Check sheet for the modelled part. Datum: model origin and axes. Units: mm. A direction names the side the tool comes from. Coordinates: 2 decimals unless noted, no trailing zeros. Loops run counter-clockwise (first coordinate to the right, second up) from the corner with the lowest first, then second, coordinate; pieces in that order, holes last. Notation, with made-up numbers: (20.25, 78) - (58.25, 78) arc R14 cw to (58.25, 103) - close; hole circle Ø1 at (-24.75, -37.5). An arc over 180 degrees is marked (long way). Write each question's results on one line, items separated by ' | '. Start each with the question number.
1. Cross-section at A-A (z = 59.5). Record the cut outline in (x, y).
2. Cross-section at B-B (y = -4.5). Record the cut outline in (x, z).
3. Draft check along X on faces 1 (the face through (-236, -11, 2)), 2 (the face through (-257, -1, 67.38)). Enter one of: released by +X, released by -X, zero draft, split by the parting line, or undercut.
4. Gauge pin test, flat end, axial feed: P1, Ø2.5, axis at x = -276.61, y = 6.8, coming from the +Z side. Record the tip position at first contact, or that the pin passes through.
5. Thickness scan on line 1 (Z direction, x = -234.5, y = -9); line 2 (Y direction, x = -240.5, z = 19); line 3 (Z direction, x = -234, y = 12). Record the ranges inside material, lowest first. Write a range as [from, to].
6. Tool access check on faces 3 (the face through (-257, -1, 0)), 4 (the face through (-257, -17.196, 33)), 5 (the face through (-235.52, 4.3, 64.37)). Record the directions out of +Z, -Z, +X, -X, +Y, -Y that give a thin tool (end or side, any length) a straight path to the whole face; none if there is none.
7. Cross-section at C-C (x = -271.5). Record the cut outline in (y, z).
```python
from build123d import *

# Parameters (mm, degrees)
SKETCH1_W               = 55.67262225
SKETCH1_H               = 40
BOSS_EXTRUDE1_DEPTH     = 4
SKETCH2_W               = 55.67262225
SKETCH2_H               = 4
BOSS_EXTRUDE2_DEPTH     = 63.38
SKETCH3_W               = 55.67262225
SKETCH3_H               = 40
BOSS_EXTRUDE3_DEPTH     = 4
SKETCH4_R               = 1.6
CUT_EXTRUDE1_DEPTH      = 64.38
CUT_EXTRUDE1_DEPTH_BACK = 5
CUT_EXTRUDE2_START      = -2
CUT_EXTRUDE2_DEPTH      = 63.38
FILLET1_R               = 3


with BuildPart() as part:
    # Sketch1 → Boss-Extrude1 (new body)
    with BuildSketch(Plane.XY):
        with Locations((-256.769960814, -1.19608299)):
            Rectangle(SKETCH1_W, SKETCH1_H)
    extrude(amount=BOSS_EXTRUDE1_DEPTH)

    # Sketch2 → Boss-Extrude2 (add)
    with BuildSketch(Plane.XY.offset(4)):
        with Locations((-256.769960814, -19.19608299)):
            Rectangle(SKETCH2_W, SKETCH2_H)
        with Locations((-256.769960814, 16.80391701)):
            Rectangle(SKETCH2_W, SKETCH2_H)
    extrude(amount=BOSS_EXTRUDE2_DEPTH)

    # Sketch3 → Boss-Extrude3 (add)
    with BuildSketch(Plane(origin=(0, 0, 67.38), x_dir=(-1, 0, 0), z_dir=(0, 0, -1))):
        with Locations((256.769960814, -1.19608299)):
            Rectangle(SKETCH3_W, SKETCH3_H)
    extrude(amount=BOSS_EXTRUDE3_DEPTH)

    # Sketch4 → Cut-Extrude1 (cut, two sides)
    with BuildSketch(Plane.XY.offset(4)) as cut_extrude1_sk:
        with Locations((-276.606271939, -9.19608299)):
            Circle(SKETCH4_R)
        with Locations((-276.606271939, 6.80391701)):
            Circle(SKETCH4_R)
        with Locations((-236.933649689, 6.80391701)):
            Circle(SKETCH4_R)
        with Locations((-236.933649689, -9.19608299)):
            Circle(SKETCH4_R)
    extrude(amount=CUT_EXTRUDE1_DEPTH, mode=Mode.SUBTRACT)
    extrude(cut_extrude1_sk.sketch, amount=-CUT_EXTRUDE1_DEPTH_BACK, mode=Mode.SUBTRACT)

    # Sketch5 → Cut-Extrude2 (cut)
    with BuildSketch(Plane.XY.offset(4).offset(CUT_EXTRUDE2_START)):
        Polygon((-276.602416628, -5.876321181), (-279.479342345, -7.532863288), (-279.483197655, -10.852625098), (-276.610127249, -12.515844799), (-273.733201533, -10.859302692), (-273.729346222, -7.539540882), align=None)
        Polygon((-276.606181369, 10.123681057), (-279.481226653, 8.463877469), (-279.481317222, 5.144113422), (-276.606362508, 3.484152963), (-273.731317224, 5.143956551), (-273.731226655, 8.463720598), align=None)
        Polygon((-236.907079951, -5.876425269), (-239.795272738, -7.513244061), (-239.821842476, -10.832901782), (-236.960219427, -12.515740711), (-234.07202664, -10.878921919), (-234.045456902, -7.559264198), align=None)
        Polygon((-236.933649689, 10.123681058), (-239.808649689, 8.463799034), (-239.808649689, 5.144034986), (-236.933649689, 3.484152962), (-234.058649689, 5.144034986), (-234.058649689, 8.463799034), align=None)
    extrude(amount=CUT_EXTRUDE2_DEPTH, mode=Mode.SUBTRACT)

    # Fillet1
    fillet1_edges = [part.edges().sort_by_distance(p)[0] for p in [
        (-256.769960814, -17.19608299, 4),
        (-256.769960814, 14.80391701, 4),
        (-256.769960814, -17.19608299, 63.38),
        (-256.769960814, 14.80391701, 63.38),
    ]]
    fillet(fillet1_edges, radius=FILLET1_R)


solid = part.part
```
Established:
1) outline: (-284.61, -21.2) - (-228.93, -21.2) - (-228.93, -17.2) - (-284.61, -17.2) - close; (-284.61, 14.8) - (-228.93, 14.8) - (-228.93, 18.8) - (-284.61, 18.8) - close
2) outline: (-284.61, 0) - (-228.93, 0) - (-228.93, 4) - (-284.61, 4) - close; (-284.61, 63.38) - (-228.93, 63.38) - (-228.93, 67.38) - (-284.61, 67.38) - close
3) face 1: undercut | face 2: zero draft
4) P1: through
5) line 1: [0, 2], [65.38, 67.38] | line 2: [-21.2, -17.2], [14.8, 18.8] | line 3: [0, 4.01], [63.37, 67.38]
6) face 3: -Z, +X, -X, +Y, -Y | face 4: +X, -X | face 5: none
7) outline: (-21.2, 0) - (18.8, 0) - (18.8, 67.38) - (-21.2, 67.38) - close; hole (-17.2, 7) arc R3 ccw to (-14.2, 4) - (11.8, 4) arc R3 ccw to (14.8, 7) - (14.8, 60.38) arc R3 ccw to (11.8, 63.38) - (-14.2, 63.38) arc R3 ccw to (-17.2, 60.38) - close
